Answer from the drawing. Dimensions are ordinates in mm from the lowest x, y and z of the part. A direction names the side the tool comes from. Coordinates: 2 decimals unless noted, no trailing zeros. Write each loop counter-clockwise with the first axis right and the second up, starting at its lowest first coordinate (ties: lowest second). Pieces come first, ordered by that corner, then holes.
(1) Given P1, Ø1.5, axis at x = 46.5, y = 31, coming from the -Z side; P2, Ø1.5, axis at x = 42, y = 55.5, coming from the +Z side (1 decimal); P3, Ø1.5, axis at x = 17, z = 88, coming from the -Y side, each flat-ended and moving along its own axis, determine where each tip first touches the part or whether it passes through.
(2) The part is cut by section A-A on y = 43. Determine the outline of the cut face in (x, z) (1 decimal), plus the area to 3 significant figures.
(3) The part is cut by section B-B on x = 65.5. Determine the outline of the cut face in (y, z) (1 decimal), plus the area to 3 significant figures.
(4) The part is cut by section C-C on z = 42.5. Determine the outline of the cut face in (x, y) (1 decimal), plus the area to 3 significant figures.
(5) Straight lines are drawn through the part: line 1 (Y direction, x = 69.5, z = 53) (1 decimal); line 2 (Z direction, x = 59.5, y = 63) (1 decimal); line 3 (X direction, y = 34, z = 68) (1 decimal). For each, find the intervals that lie inside material, in ascending order.
(6) For a pull along X with two mould halves and no side action, classify the marked faces 1, 2 and 3 as +X half, -X half, draft (parallel to the pull), parting line (faces both ways), or undercut.
(7) The part is cut by section D-D on y = 26. Determine the outline of the cut face in (x, z) (1 decimal).
(8) Which of the six approach directions +Z, -Z, +X, -X, +Y, -Y give full straight-line access (tool end or side, diameter ignored) to the marked faces 4 and 5?
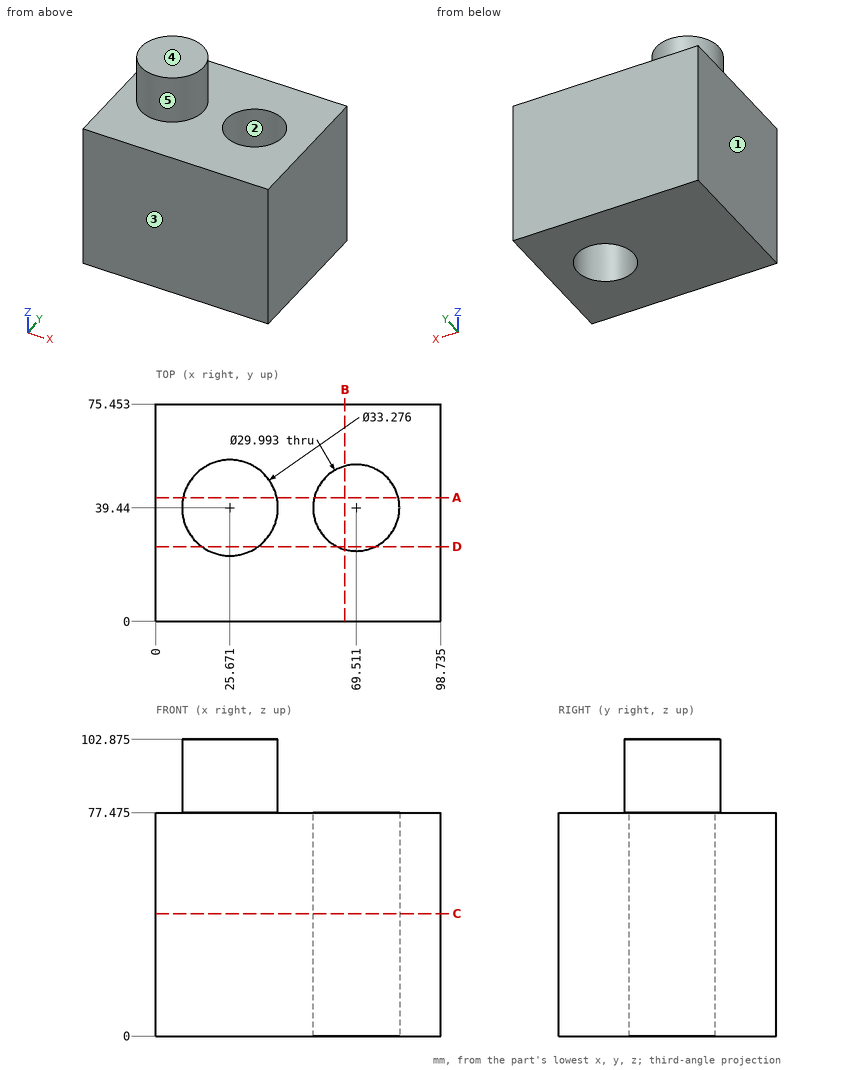
Model answer:
1. P1: stops at z = 0
1. P2: stops at z = 77.5
1. P3: stops at y = 24.81
2. outline: (0, 0) - (54.9, 0) - (54.9, 77.5) - (41.9, 77.5) - (41.9, 102.9) - (9.4, 102.9) - (9.4, 77.5) - (0, 77.5) - close; (84.1, 0) - (98.7, 0) - (98.7, 77.5) - (84.1, 77.5) - close
2. area: 6,220 mm2
3. outline: (0, 0) - (25, 0) - (25, 77.5) - (0, 77.5) - close; (53.9, 0) - (75.5, 0) - (75.5, 77.5) - (53.9, 77.5) - close
3. area: 3,610 mm2
4. outline: (0, 0) - (98.7, 0) - (98.7, 75.5) - (0, 75.5) - close; hole circle Ø30 at (69.5, 39.4)
4. area: 6,740 mm2
5. line 1: y = 0 to 24.4, 54.4 to 75.5
5. line 2: z = 0 to 77.5
5. line 3: x = 0 to 55.5, 83.5 to 98.7
6. face 1: -X half
6. face 2: undercut
6. face 3: draft
7. outline: (0, 0) - (62.9, 0) - (62.9, 77.5) - (35.5, 77.5) - (35.5, 102.9) - (15.9, 102.9) - (15.9, 77.5) - (0, 77.5) - close; (76.2, 0) - (98.7, 0) - (98.7, 77.5) - (76.2, 77.5) - close
8. face 4: +Z, +X, -X, +Y, -Y
8. face 5: +Z
